Input: dimensioned drawing with shaded views. Units: mm. Origin: part minimum x, y, z. Give positions to 0.01 mm unless a question says otherwise; leave off trailing zeros. Order: outer loops, then holes, each group sorted by start corner. A loop starts at its lowest first (then second) coordinate and runs counter-clockwise, first axis right, second up. Notation, with made-up numbers: (54, 68) -> (71, 68) arc R27 cw to (71, 103) -> close; hole circle Ø11 at (7.25, 82.25). An arc over 180 degrees is marked (long way). One line per question, with ' | ' between items. Start each with the question number.
(1) Section D-D (y = 55). Return loops of the section in (x, z), then the cut area to 3 significant figures.
(2) Section C-C (z = 2.25). Return loops of the section in (x, y), then the cut area to 3 significant figures.
(3) Ray query, L1, parallel to Y at x = 7, z = 1.85; L2, parallel to Y at x = 28.5, z = 0.4; L3, parallel to X at y = 37.5, z = 2.6. Return the intervals inside material, ascending.
(4) First-contact query: pin 1 Ø2 at (x, y) = (7, 55) entering from -Z. Flat tip, straight axial feed; report the tip coordinate or a pass-through.
(5) Mould query, pull axis Z, two halves, no side actions, for the marked faces 1 and 2. Classes: +Z half, -Z half, draft (parallel to the pull), parting line (faces both ways), or undercut.
(6) Section B-B (y = 30.5). Return loops of the section in (x, z), then the cut area to 3 significant figures.
(7) Section A-A (x = 22.5). Return loops of the section in (y, z), then the cut area to 3 significant figures.
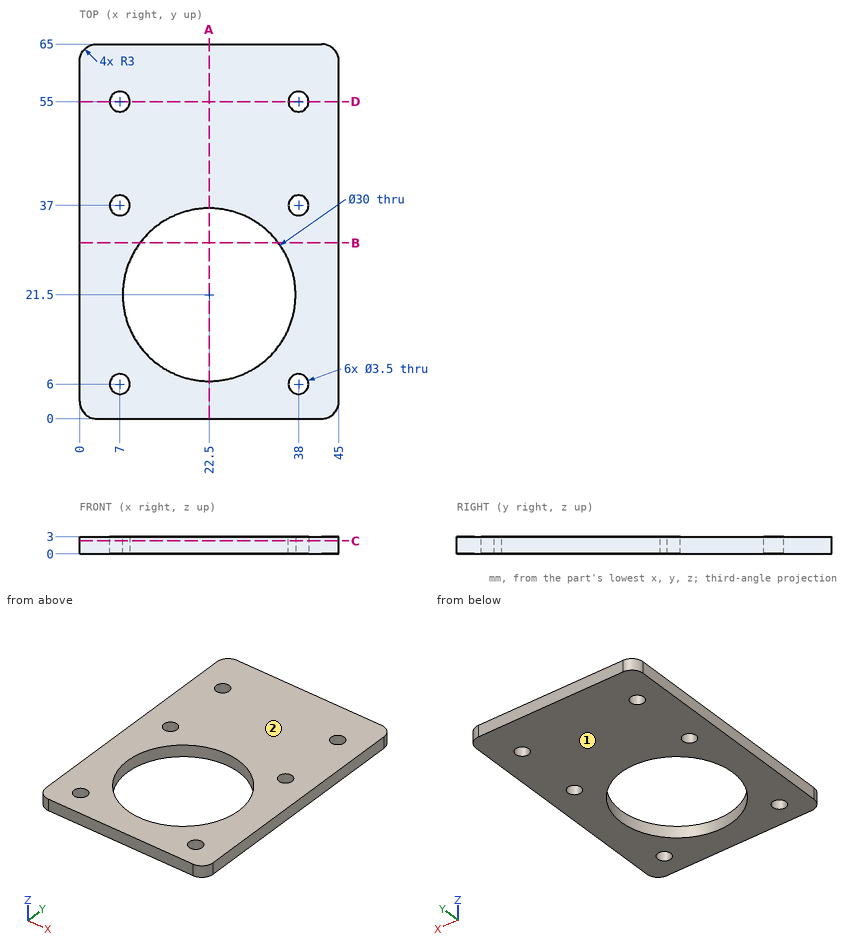
Response:
1) outline: (0, 0) -> (5.25, 0) -> (5.25, 3) -> (0, 3) -> close; (8.75, 0) -> (36.25, 0) -> (36.25, 3) -> (8.75, 3) -> close; (39.75, 0) -> (45, 0) -> (45, 3) -> (39.75, 3) -> close | area: 114 mm^2
2) outline: (0, 3) arc R3 ccw to (3, 0) -> (42, 0) arc R3 ccw to (45, 3) -> (45, 62) arc R3 ccw to (42, 65) -> (3, 65) arc R3 ccw to (0, 62) -> close; hole circle Ø3.5 at (7, 6); hole circle Ø3.5 at (7, 37); hole circle Ø3.5 at (7, 55); hole circle Ø30 at (22.5, 21.5); hole circle Ø3.5 at (38, 6); hole circle Ø3.5 at (38, 37); hole circle Ø3.5 at (38, 55) | area: 2,150 mm^2
3) L1: y = 0 to 4.25, 7.75 to 35.25, 38.75 to 53.25, 56.75 to 65 | L2: y = 0 to 7.75, 35.25 to 65 | L3: x = 0 to 5.32, 8.68 to 36.32, 39.68 to 45
4) pin 1: passes through
5) face 1: -Z half | face 2: +Z half
6) outline: (0, 0) -> (10.5, 0) -> (10.5, 3) -> (0, 3) -> close; (34.5, 0) -> (45, 0) -> (45, 3) -> (34.5, 3) -> close | area: 63.0 mm^2
7) outline: (0, 0) -> (6.5, 0) -> (6.5, 3) -> (0, 3) -> close; (36.5, 0) -> (65, 0) -> (65, 3) -> (36.5, 3) -> close | area: 105 mm^2
